from build123d import *

# Parameters (mm, degrees)
SKETCH1_W           = 248.92
SKETCH1_H           = 106.68
BOSS_EXTRUDE1_DEPTH = 50.8
SKETCH2_W           = 177.8
SKETCH2_H           = 106.68
CUT_EXTRUDE1_DEPTH  = 15.24
SKETCH3_R           = 15.24
CUT_EXTRUDE3_DEPTH  = 35.56
SKETCH3_4_W         = 35.56
SKETCH3_4_H         = 106.68
BOSS_EXTRUDE2_DEPTH = 106.68
SKETCH4_R           = 25.4
CUT_EXTRUDE4_DEPTH  = 35.56
FILLET1_R           = 53.34
FILLET2_R           = 12.7
FILLET3_R           = 12.7


with BuildPart() as part:
    # Sketch1 → Boss-Extrude1 (new body)
    with BuildSketch(Plane(origin=(0, 0, 0), x_dir=(1, 0, 0), z_dir=(0, 1, 0))):
        with Locations((124.46, -53.34)):
            Rectangle(SKETCH1_W, SKETCH1_H)
    extrude(amount=BOSS_EXTRUDE1_DEPTH)

    # Sketch2 → Cut-Extrude1 (cut)
    with BuildSketch(Plane.XZ):
        with Locations((124.46, 53.34)):
            Rectangle(SKETCH2_W, SKETCH2_H)
    extrude(amount=-CUT_EXTRUDE1_DEPTH, mode=Mode.SUBTRACT)

    # Sketch3 → Cut-Extrude3 (cut)
    with BuildSketch(Plane(origin=(0, 50.8, 0), x_dir=(1, 0, 0), z_dir=(0, 1, 0))):
        with Locations(Location((60.96, -53.34, 0), (0, 0, 270))):
            Circle(SKETCH3_R)
        with Locations(Location((187.96, -53.34, 0), (0, 0, 270))):
            Circle(SKETCH3_R)
    extrude(amount=-CUT_EXTRUDE3_DEPTH, mode=Mode.SUBTRACT)

    # Sketch3<4> → Boss-Extrude2 (add)
    with BuildSketch(Plane(origin=(0, 50.8, 0), x_dir=(1, 0, 0), z_dir=(0, 1, 0))):
        with Locations((124.46, -53.34)):
            Rectangle(SKETCH3_4_W, SKETCH3_4_H)
    extrude(amount=BOSS_EXTRUDE2_DEPTH)

    # Sketch4 → Cut-Extrude4 (cut)
    with BuildSketch(Plane(origin=(142.24, 0, 0), x_dir=(0, 0, -1), z_dir=(1, 0, 0))):
        with Locations((-53.34, 104.14)):
            Circle(SKETCH4_R)
    extrude(amount=-CUT_EXTRUDE4_DEPTH, mode=Mode.SUBTRACT)

    # Fillet1
    fillet1_edges = [part.edges().sort_by_distance(p)[0] for p in [
        (124.46, 157.48, 106.68),
        (124.46, 157.48, 0),
    ]]
    fillet(fillet1_edges, radius=FILLET1_R - 0.0001)  # a hair under: the kernel refuses the full size

    # Fillet2
    fillet2_edges = [part.edges().sort_by_distance(p)[0] for p in [
        (248.92, 50.8, 53.34),
        (0, 50.8, 53.34),
    ]]
    fillet(fillet2_edges, radius=FILLET2_R)

    # Fillet3
    fillet3_edges = [part.edges().sort_by_distance(p)[0] for p in [
        (106.68, 50.8, 53.34),
        (142.24, 50.8, 53.34),
    ]]
    fillet(fillet3_edges, radius=FILLET3_R)


solid = part.part
CAD build for the part. Positions are in the model's coordinates, mm. A direction names the side the tool comes from. Give positions to 0.01 mm unless a question says otherwise; leave off trailing zeros. Order: outer loops, then holes, each group sorted by start corner. A loop starts at its lowest first (then second) coordinate and runs counter-clockwise, first axis right, second up. Notation, with made-up numbers: (1, 58.5) - (5, 58.5) arc R17 cw to (5, 73.5) - close; hole circle Ø1 at (76, 24). An arc over 180 degrees is marked (long way). Write each question's results on one line, items separated by ' | '.
1. Saw through at A-A on x = 187.96. List the corners of the cut face in (y, z).
Calculated:
outline: (15.24, 0) - (50.8, 0) - (50.8, 38.1) - (15.24, 38.1) - close; (15.24, 68.58) - (50.8, 68.58) - (50.8, 106.68) - (15.24, 106.68) - close
2. Saw through at D-D on x = 84. List the corners of the cut face in (y, z), and give its area (3 significant figures).
Calculated:
outline: (15.24, 0) - (50.8, 0) - (50.8, 106.68) - (15.24, 106.68) - close | area: 3,790 mm2
3. Saw through at C-C on z = 74. List the corners of the cut face in (x, y).
Calculated:
outline: (0, 0) - (35.56, 0) - (35.56, 15.24) - (213.36, 15.24) - (213.36, 0) - (248.92, 0) - (248.92, 38.1) arc R12.7 ccw to (236.22, 50.8) - (154.94, 50.8) arc R12.7 cw to (142.24, 63.5) - (142.24, 89.36) - (106.68, 89.36) - (106.68, 63.5) arc R12.7 cw to (93.98, 50.8) - (12.7, 50.8) arc R12.7 ccw to (0, 38.1) - close; (106.68, 118.92) - (142.24, 118.92) - (142.24, 153.32) - (106.68, 153.32) - close
4. Probe L1, parallel to X at y = 36, z = 53; L2, parallel to Y at x = 129.5, z = 53.34; L3, parallel to Z at x = 116, y = 104. List the from-to ranges inside material, lowest first. Write a range as from..to.
Calculated:
L1: x = 0..45.72, 76.2..172.72, 203.2..248.92 | L2: y = 15.24..78.74, 129.54..157.48 | L3: z = 0..27.94, 78.74..106.68
5. 3-axis set-ups, long thin cutter, end or side, ignore diameter. For faces 1 (the face through (204, 50.8, 53)), 2 (the face through (213.36, 8, 53)), 3 (the face through (44, 50.8, 53)): which of +Z, -Z, +X, -X, +Y, -Y reach the whole face in a straight line?
Calculated:
face 1: +Z, -Z, +X, +Y | face 2: +Z, -Z, -Y | face 3: +Z, -Z, -X, +Y
6. Saw through at B-B on y = 94. List the corners of the cut face in (x, z), and give its area (3 significant figures).
Calculated:
outline: (106.68, 0) - (142.24, 0) - (142.24, 30.05) - (106.68, 30.05) - close; (106.68, 76.63) - (142.24, 76.63) - (142.24, 106.68) - (106.68, 106.68) - close | area: 2,140 mm2
7. Pull direction Z, two halves, no side cores. Call faces 4 (the face through (174.44, 33.27, 60.37)), 5 (the face through (123, 40, 106.68)), 6 (the face through (76.07, 33.27, 51.36)), 7 (the face through (35.56, 8, 53)): released by +Z, released by -Z, zero draft, split by the parting line, or undercut.
Calculated:
face 4: undercut | face 5: released by +Z | face 6: undercut | face 7: zero draft
8. Pin check, flat tips, straight feed: pin 1 (24.5 mm diameter, centred on x = 188, z = 40, fed in from +Y); pin 2 (6 mm diameter, centred on y = 87.5, z = 92.5, fed in from -X); pin 3 (12 mm diameter, centred on x = 138, z = 84.5, fed in from +Y). Stop position of each tip, or through.
Calculated:
pin 1: stops at y = 50.8 | pin 2: stops at x = 106.68 | pin 3: stops at y = 151.17
